```python
from build123d import *

# Parameters (mm, degrees)
SKETCH1_R           = 1.8288
BOSS_EXTRUDE1_DEPTH = 6.35


with BuildPart() as part:
    # Sketch1 → Boss-Extrude1 (new body)
    with BuildSketch(Plane(origin=(0, 0, 0), x_dir=(1, 0, 0), z_dir=(0, 1, 0))):
        Polygon((-48.0314, 88.9), (48.0314, 88.9), (48.0314, 73.152), (-15.4686, 73.152), (-15.4686, 66.548), (48.0314, 66.548), (48.0314, 35.052), (-15.4686, 35.052), (-15.4686, 28.448), (48.0314, 28.448), (48.0314, -3.048), (-15.4686, -3.048), (-15.4686, -9.652), (48.0314, -9.652), (48.0314, -41.148), (-15.4686, -41.148), (-15.4686, -47.752), (48.0314, -47.752), (48.0314, -88.9), (-48.0314, -88.9), (-48.0314, -27.2288), (-44.3484, -27.2288), (-44.3484, -29.337), (-41.6814, -29.337), (-41.6814, -21.463), (-44.3484, -21.463), (-44.3484, -23.5712), (-48.0314, -23.5712), (-48.0314, 10.8712), (-44.3484, 10.8712), (-44.3484, 8.763), (-41.6814, 8.763), (-41.6814, 16.637), (-44.3484, 16.637), (-44.3484, 14.5288), (-48.0314, 14.5288), (-48.0314, 48.9712), (-44.3484, 48.9712), (-44.3484, 46.863), (-41.6814, 46.863), (-41.6814, 54.737), (-44.3484, 54.737), (-44.3484, 52.6288), (-48.0314, 52.6288), align=None)
        with Locations((-38.1, 69.85)):
            Circle(SKETCH1_R, mode=Mode.SUBTRACT)
        with Locations((-38.1, 31.75)):
            Circle(SKETCH1_R, mode=Mode.SUBTRACT)
        with Locations((-38.1, -6.35)):
            Circle(SKETCH1_R, mode=Mode.SUBTRACT)
        with Locations((-38.1, -44.45)):
            Circle(SKETCH1_R, mode=Mode.SUBTRACT)
    extrude(amount=-BOSS_EXTRUDE1_DEPTH)


solid = part.part
```
Could you check a few things on this model? Use its own coordinates, in mm. A direction names the side the tool comes from. Round coordinates to 2 decimals unless told otherwise and drop trailing zeros. Order: outer loops, then holes, each group sorted by start corner. A loop starts at its lowest first (then second) coordinate and runs counter-clockwise, first axis right, second up. Notation, with made-up numbers: (-15, 38.5) -> (11, 38.5) arc R30 cw to (11, 75.5) -> close; hole circle Ø8 at (-15, -31.75). An arc over 180 degrees is marked (long way). One line per question, with ' | ' between items.
Q1. Which directions (+Z, -Z, +X, -X, +Y, -Y) give clear straight access to the entire face, cutting with the end or side of a thin tool? Please do faces 4 (the face through (-41.681, -3, 25)), 5 (the face through (-46, -3, -14.529)), 6 (the face through (-48.031, -3, 7)), 7 (the face through (16, -3, -66.548)).
Computed values:
face 4: +Y, -Y | face 5: -X, +Y, -Y | face 6: +Z, -Z, -X, +Y, -Y | face 7: +X, +Y, -Y
Q2. I'm going to push flat-ended pins straight in: pin 1 (2 mm diameter, centred on x = -38.1, z = 6.35, fed in from +Y); pin 2 (1.9 mm diameter, centred on y = -4, z = 5, fed in from +X). Where does each tip first touch, or does it pass through?
Computed values:
pin 1: through | pin 2: x = -15.47
Q3. If we section it at C-C on x = -38.1: Write out the boundary of the cut face in (y, z), plus the area to 3 significant figures.
Computed values:
outline: (-6.35, -88.9) -> (0, -88.9) -> (0, -71.68) -> (-6.35, -71.68) -> close; (-6.35, -68.02) -> (0, -68.02) -> (0, -33.58) -> (-6.35, -33.58) -> close; (-6.35, -29.92) -> (0, -29.92) -> (0, 4.52) -> (-6.35, 4.52) -> close; (-6.35, 8.18) -> (0, 8.18) -> (0, 42.62) -> (-6.35, 42.62) -> close; (-6.35, 46.28) -> (0, 46.28) -> (0, 88.9) -> (-6.35, 88.9) -> close | area: 1,040 mm²
Q4. If we section it at D-D on y = -4.5: Give the number of separate pieces and of enclosed holes in the cut face, plus the area to 3 significant figures.
Computed values:
separate pieces: 1 | enclosed holes: 4 | area: 15,300 mm²
Q5. If we section it at B-B on z = -69.85: Write out the boundary of the cut face in (x, y), plus the area to 3 significant figures.
Computed values:
outline: (-48.03, -6.35) -> (-39.93, -6.35) -> (-39.93, 0) -> (-48.03, 0) -> close; (-36.27, -6.35) -> (-15.47, -6.35) -> (-15.47, 0) -> (-36.27, 0) -> close | area: 184 mm²
Q6. If we section it at A-A on x = -5.5: Write out the boundary of the cut face in (y, z).
Computed values:
outline: (-6.35, -88.9) -> (0, -88.9) -> (0, -73.15) -> (-6.35, -73.15) -> close; (-6.35, -66.55) -> (0, -66.55) -> (0, -35.05) -> (-6.35, -35.05) -> close; (-6.35, -28.45) -> (0, -28.45) -> (0, 3.05) -> (-6.35, 3.05) -> close; (-6.35, 9.65) -> (0, 9.65) -> (0, 41.15) -> (-6.35, 41.15) -> close; (-6.35, 47.75) -> (0, 47.75) -> (0, 88.9) -> (-6.35, 88.9) -> close
Q7. If I drill on line 1 (Z direction, x = -38.1, y = -3.75); line 2 (Z direction, x = 38.5, y = -0.75); line 3 (X direction, y = -2.25, z = 44.45), over which ranges is the centre line in solid material (lowest first)? Write a range as from..to.
Computed values:
line 1: -88.9..-71.68, -68.02..-33.58, -29.92..4.52, 8.18..42.62, 46.28..88.9 | line 2: -88.9..-73.15, -66.55..-35.05, -28.45..3.05, 9.65..41.15, 47.75..88.9 | line 3: -48.03..-39.93, -36.27..-15.47
Q8. We'd pull the mould along Z, two halves only. Please class faces 1 (the face through (1, -3, 88.9)), 2 (the face through (-48.031, -3, -71)), 3 (the face through (-46, -3, 27.229)): released by +Z, released by -Z, zero draft, split by the parting line, or undercut.
Computed values:
face 1: released by +Z | face 2: zero draft | face 3: undercut
